Model file for the job. Use its own axes, mm. A direction names the side the tool comes from. Round coordinates to 2 decimals unless told otherwise and drop trailing zeros. Order: outer loops, then holes, each group sorted by start corner. A loop starts at its lowest first (then second) coordinate and runs counter-clockwise, first axis right, second up. Notation, with made-up numbers: (-15.75, -25.75) -> (-6.75, -25.75) arc R23 cw to (-6.75, -2.75) -> close; hole circle Ø7 at (-22.5, 36). An arc over 180 degrees is marked (long way). Answer as CSV lines item,"result".
```python
from build123d import *

# Parameters (mm, degrees)
PROFILESKETCH1_W                          = 4
PROFILESKETCH1_H                          = 58.1
BOSS_EXTRUDE1_DEPTH                       = 26
PROBESLIDINGMOUNTSKETCH4_R                = 1.55
PROBESLIDINGMOUNTCUT_EXTRUDE3_DEPTH       = 64.77781746
PROBESLIDINGMOUNTCHANELCUT_EXTRUDE4_DEPTH = 1
INDUCTIVEPROBEHOLDERSKETCH1_W             = 4.15
INDUCTIVEPROBEHOLDERSKETCH1_H             = 25
INDUCTIVEPROBEHOLDERBOSS_EXTRUDE2_DEPTH   = 17.8


with BuildPart() as part:
    # ProfileSketch1 → Boss-Extrude1 (new body)
    with BuildSketch(Plane.XY):
        with Locations((2, 29.05)):
            Rectangle(PROFILESKETCH1_W, PROFILESKETCH1_H)
    extrude(amount=BOSS_EXTRUDE1_DEPTH)

    # ProbeSlidingMountSketch4 → ProbeSlidingMountCut-Extrude3 (cut, through all)
    with BuildSketch(Plane.ZY):
        with Locations(Location((7.2, 16.5, 0), (0, 0, 270))):
            Circle(PROBESLIDINGMOUNTSKETCH4_R)
        with Locations(Location((18.8, 16.5, 0), (0, 0, 270))):
            Circle(PROBESLIDINGMOUNTSKETCH4_R)
        with BuildLine():
            Line((5.65, 49.9), (5.65, 40.9))
            ThreePointArc((5.65, 40.9), (7.2, 39.35), (8.75, 40.9))
            Line((8.75, 40.9), (8.75, 49.9))
            ThreePointArc((8.75, 49.9), (7.2, 51.45), (5.65, 49.9))
        make_face()
        with BuildLine():
            Line((17.25, 49.9), (17.25, 40.9))
            ThreePointArc((17.25, 40.9), (18.8, 39.35), (20.35, 40.9))
            Line((20.35, 40.9), (20.35, 49.9))
            ThreePointArc((20.35, 49.9), (18.8, 51.45), (17.25, 49.9))
        make_face()
    extrude(amount=-PROBESLIDINGMOUNTCUT_EXTRUDE3_DEPTH, mode=Mode.SUBTRACT)

    # ProbeSlidingMountChannelSketch5 → ProbeSlidingMountChanelCut-Extrude4 (cut)
    with BuildSketch(Plane.ZY):
        with BuildLine():
            Line((10.4, 49.9), (10.4, 40.9))
            ThreePointArc((10.4, 40.9), (7.2, 37.7), (4, 40.9))
            Line((4, 40.9), (4, 49.9))
            ThreePointArc((4, 49.9), (7.2, 53.1), (10.4, 49.9))
        make_face()
        with BuildLine():
            Line((22, 49.9), (22, 40.9))
            ThreePointArc((22, 40.9), (18.8, 37.7), (15.6, 40.9))
            Line((15.6, 40.9), (15.6, 49.9))
            ThreePointArc((15.6, 49.9), (18.8, 53.1), (22, 49.9))
        make_face()
    extrude(amount=-PROBESLIDINGMOUNTCHANELCUT_EXTRUDE4_DEPTH, mode=Mode.SUBTRACT)

    # InductiveProbeHolderSketch1 → InductiveProbeHolderBoss-Extrude2 (add)
    with BuildSketch(Plane.ZY):
        with Locations((2.075, 12.5)):
            Rectangle(INDUCTIVEPROBEHOLDERSKETCH1_W, INDUCTIVEPROBEHOLDERSKETCH1_H)
        with Locations((23.925, 12.5)):
            Rectangle(INDUCTIVEPROBEHOLDERSKETCH1_W, INDUCTIVEPROBEHOLDERSKETCH1_H)
    extrude(amount=INDUCTIVEPROBEHOLDERBOSS_EXTRUDE2_DEPTH)


solid = part.part
```
Q1. Wall check: L1, parallel to Z at x = 1.25, y = 16.5; L2, parallel to Z at x = -6.5, y = 15.5; L3, parallel to Y at x = -3, z = 4. Give the ranges that are in metal, low to high. Write a range as [from, to].
Checks:
L1,"[0, 5.65], [8.75, 17.25], [20.35, 26]"
L2,"[0, 4.15], [21.85, 26]"
L3,"[0, 25]"
Q2. Saw through at B-B (z = 7.2). Write the cut outline in (x, y), plus the area to 3 significant figures.
Checks:
outline,"(0, 0) -> (4, 0) -> (4, 14.95) -> (0, 14.95) -> close; (0, 18.05) -> (4, 18.05) -> (4, 39.35) -> (1, 39.35) -> (1, 37.7) -> (0, 37.7) -> close; (0, 53.1) -> (1, 53.1) -> (1, 51.45) -> (4, 51.45) -> (4, 58.1) -> (0, 58.1) -> close"
area,"168 mm²"
Q3. Flat gauge pins, fed straight in: pin 1 (5 mm diameter, centred on y = 49, z = 8.5, fed in from -X); pin 2 (2 mm diameter, centred on x = -4.5, z = 23, fed in from +Y); pin 3 (3 mm diameter, centred on y = 42, z = 19, fed in from -X). Where does each tip first touch, or does it go through?
Checks:
pin 1,"x = 0"
pin 2,"y = 25"
pin 3,"x = 1"
Q4. Saw through at C-C (x = -1.75). Write the cut outline in (y, z).
Checks:
outline,"(0, 0) -> (25, 0) -> (25, 4.15) -> (0, 4.15) -> close; (0, 21.85) -> (25, 21.85) -> (25, 26) -> (0, 26) -> close"
Q5. Tool access for faces 1 (the flat face through (-9, 12, 21.85)), 2 (the cylindrical face through (0.5, 53.1, 18.7)), 3 (the cylindrical face through (2.48, 51.45, 18.83)), 4 (the flat face through (-9, 25, 2)): list every direction of +Z, -Z, +X, -X, +Y, -Y with a clear straight run to the whole face (end or side of a thin tool).
Checks:
face 1,"-X, +Y, -Y"
face 2,"-X"
face 3,"+X, -X"
face 4,"+Z, -Z, -X, +Y"
Q6. Saw through at D-D (x = 2.75). Write the cut outline in (y, z).
Checks:
outline,"(0, 0) -> (58.1, 0) -> (58.1, 26) -> (0, 26) -> close; hole circle Ø3.1 at (16.5, 7.2); hole circle Ø3.1 at (16.5, 18.8); hole (40.9, 5.65) -> (49.9, 5.65) arc R1.55 ccw to (49.9, 8.75) -> (40.9, 8.75) arc R1.55 ccw to start; hole (40.9, 17.25) -> (49.9, 17.25) arc R1.55 ccw to (49.9, 20.35) -> (40.9, 20.35) arc R1.55 ccw to start"
Q7. Saw through at A-A (y = 16.5). Write the cut outline in (x, z).
Checks:
outline,"(-17.8, 0) -> (4, 0) -> (4, 5.65) -> (0, 5.65) -> (0, 4.15) -> (-17.8, 4.15) -> close; (-17.8, 21.85) -> (0, 21.85) -> (0, 20.35) -> (4, 20.35) -> (4, 26) -> (-17.8, 26) -> close; (0, 8.75) -> (4, 8.75) -> (4, 17.25) -> (0, 17.25) -> close"
